```python
from build123d import *

# Parameters (mm, degrees)
CARD_W              = 215
CARD_H              = 107.4
BOSS_EXTRUDE1_DEPTH = 1.5
SKETCH2_W           = 119.2
SKETCH2_H           = 39
BOSS_EXTRUDE2_DEPTH = 1
SKETCH3_W           = 1
SKETCH3_H           = 39
BOSS_EXTRUDE3_DEPTH = 11.7
BOSS_EXTRUDE4_DEPTH = 35


with BuildPart() as part:
    # card → Boss-Extrude1 (new body)
    with BuildSketch(Plane(origin=(0, 0, 0), x_dir=(1, 0, 0), z_dir=(0, 1, 0))):
        with Locations((107.5, 53.7)):
            Rectangle(CARD_W, CARD_H)
    extrude(amount=BOSS_EXTRUDE1_DEPTH)

    # Sketch2 → Boss-Extrude2 (add)
    with BuildSketch(Plane(origin=(215, 0, 0), x_dir=(0, 0, -1), z_dir=(1, 0, 0))):
        with Locations((75.8, -18)):
            Rectangle(SKETCH2_W, SKETCH2_H)
    extrude(amount=BOSS_EXTRUDE2_DEPTH)

    # Sketch3 → Boss-Extrude3 (add)
    with BuildSketch(Plane(origin=(216, 0, 0), x_dir=(0, 0, -1), z_dir=(1, 0, 0))):
        with Locations((16.7, -18)):
            Rectangle(SKETCH3_W, SKETCH3_H)
    extrude(amount=BOSS_EXTRUDE3_DEPTH)

    # Sketch5 → Boss-Extrude4 (add)
    with BuildSketch(Plane.XZ):
        Polygon((213, 0), (213, -107.4), (0, -107.4), (-12.5, -102.4), (-17, -53.7), (-12.5, -5), (0, 0.14109814), (213, 0.14109814), align=None)
    extrude(amount=BOSS_EXTRUDE4_DEPTH)


solid = part.part
```
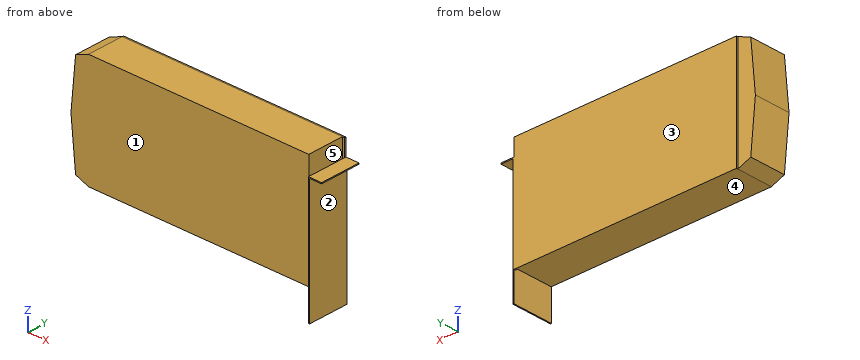
Part model, mm, in its own coordinate system. Face numbers are marked on the shaded views. A direction names the side the tool comes from. Give positions to 0.01 mm unless a question says otherwise; leave off trailing zeros. Loops run counter-clockwise (first coordinate to the right, second up) from the corner with the lowest first, then second, coordinate; pieces in that order, holes last. Notation, with made-up numbers: M 62,57 L 67,57 A31 cw 67,94 Z; hole C 14,3.25 d1. An arc over 180 degrees is marked long. Return JSON: item names as keys, results as strings.
1) Saw through at D-D, the plane z = -57.5. List the corners of the cut face in (x, y), then the cut area to 3 significant figures.
Calculated:
{"outline": "M -16.65,-35 L 213,-35 L 213,0 L 215,0 L 215,-37.5 L 216,-37.5 L 216,1.5 L 0,1.5 L 0,0 L -16.65,0 Z", "area": "8,400 mm2"}
2) 3-axis set-ups, long thin cutter, end or side, ignore diameter. For the marked faces 1, 2, 3, 4 and 5: which of +Z, -Z, +X, -X, +Y, -Y reach the whole face in a straight line?
Calculated:
{"face 1": "+Z, -Z, -X, -Y", "face 2": "-Z, +X, +Y, -Y", "face 3": "+Z, -Z, +X, -X, +Y", "face 4": "-Z, -X, +Y, -Y", "face 5": "+Z, -Z, -Y"}
3) Flat gauge pins, fed straight in: pin 1 Ø2 at (y, z) = (-9.5, -50) entering from -X; pin 2 Ø5 at (x, y) = (122, -25.5) entering from -Z; pin 3 Ø3.5 at (x, y) = (223, -17.5) entering from -Z. Where does each tip first touch, or does it go through?
Calculated:
{"pin 1": "stops at x = -16.75", "pin 2": "stops at z = -107.4", "pin 3": "stops at z = -17.2"}
4) Saw through at A-A, the plane y = -13. List the corners of the cut face in (x, z), then the cut area to 3 significant figures.
Calculated:
{"outline": "M -17,-53.7 L -12.5,-102.4 L 0,-107.4 L 213,-107.4 L 213,0.14 L 0,0.14 L -12.5,-5 Z; M 215,-135.4 L 216,-135.4 L 216,-17.2 L 227.7,-17.2 L 227.7,-16.2 L 215,-16.2 Z", "area": "24,500 mm2"}
5) Saw through at B-B, the plane x = 190.5. List the corners of the cut face in (y, z).
Calculated:
{"outline": "M -35,-107.4 L 1.5,-107.4 L 1.5,0 L 0,0 L 0,0.14 L -35,0.14 Z"}
6) Saw through at C-C, the plane z = -78. List the corners of the cut face in (x, y).
Calculated:
{"outline": "M -14.75,-35 L 213,-35 L 213,0 L 215,0 L 215,-37.5 L 216,-37.5 L 216,1.5 L 0,1.5 L 0,0 L -14.75,0 Z"}
7) Drill centre lines: line 1 (Z direction, x = 69, y = -8.5); line 2 (X direction, y = -3.5, z = -22.5); line 3 (Y direction, x = 138, z = -18.5). Where is each one in solid material? Low to high.
Calculated:
{"line 1": "z = -107.4 to 0.14", "line 2": "x = -14.12 to 213, 215 to 216", "line 3": "y = -35 to 1.5"}
